Could you check a few things on this model? Use its own coordinates, in mm. A direction names the side the tool comes from. Coordinates: 2 decimals unless noted, no trailing zeros. Write each loop counter-clockwise with the first axis right and the second up, starting at its lowest first coordinate (ties: lowest second). Pieces come first, ordered by that corner, then holes.
Item 1: I want a section at C-C on x = -6.5. Please give me the cut outline in (y, z).
Item 2: Thinking about a two-plate mould opening in Z: for faces 1 (the cylindrical face through (0.18, 148.5, 0.07)), 2 (the flat face through (0, 160, 0)), 3 (the cylindrical face through (-11.923, 78.88, -3.755)), which applies, +Z half, -Z half, draft (parallel to the pull), parting line (faces both ways), or undercut?
Item 3: Which directions (+Z, -Z, +X, -X, +Y, -Y) give clear straight access to the entire face, cutting with the end or side of a thin tool? Please do faces 4 (the cylindrical face through (-0.05, 4.06, -3.77)), 5 (the flat face through (0, 0, 0)).
Item 4: I want a section at A-A on z = 0. Please give me the cut outline in (x, y), then the cut area to 3 significant figures.
Item 5: For P1, Ø2, axis at x = 0, z = -5, coming from the -Y side; P2, Ø1, axis at y = 114.5, z = 6.5, coming from the +X side; P3, Ø2, axis at y = 83.5, z = 2.5, coming from the +X side, each with a flat end and sliding along its axis, tell me the tip position at first contact or that it passes through.
Item 6: I want a section at D-D on z = 8. Please give me the cut outline in (x, y), then the cut area to 3 significant figures.
Item 7: I want a section at B-B on y = 55. Please give me the cut outline in (x, z), then the cut area to 3 significant figures.
Item 8: If I drill on probe 1 along Z at (x, y) = (0, 4.75); probe 2 along Y at (x, z) = (2.25, 0); probe 3 along Y at (x, z) = (-6.25, -1), over which ranges is the centre line in solid material (lowest first)?
Autodesk Inventor part; units mm, degrees
ref_plane "YZ Plane" through (0, 0, 0) normal (1, 0, 0) x (0, 1, 0)
ref_plane "XZ Plane" through (0, 0, 0) normal (0, 1, 0) x (-1, 0, 0)
ref_plane "XY Plane" through (0, 0, 0) normal (0, 0, 1) x (1, 0, 0)
sketch "Эскиз1" plane through (0, 0, 0) normal (0, 1, 0) x (-1, 0, 0)
  circle A0 centre (0, 0) radius 12.5
  dimension "d0" = 25
extrude "Выдавливание1" add sketch "Эскиз1" along normal blind 160
sketch "Эскиз2" plane through (0, 0, 0) normal (0, -1, 0) x (1, 0, 0)
  circle A0 centre (0, 0) radius 22.5
  line L0 (0, 0) -> (0, 5)
  line L1 (0, 0) -> (0, -5)
  dimension "d3" = 45
  dimension "d4" = 5
  dimension "d5" = 5
hole "Отверстие1" at (0, 0, 5) at (0, 0, -5) direction (0, 1, 0) diameter 2.459 depth 8 tip angle 118
sketch "Эскиз4" plane through (0, 0, 0) normal (1, 0, 0) x (0, 1, 0)
  line L0 (160, -12.5) -> (160, 12.5)
  line L1 (160, 0) -> (150, 0)
  circle A0 centre (150, 0) radius 1.5
  line L2 (160, 0) -> (150, 0)
  line L3 (150, 0) -> (155, 0)
  circle A1 centre (145, 0) radius 1.5
  line L4 (0, 0) -> (50, 0)
  circle A2 centre (50, 0) radius 1.5
  dimension "d30" = 3
  dimension "d35" = 10
  dimension "d49" = 50
  dimension "d50" = 3
extrude "Выдавливание3" cut sketch "Эскиз4" along normal mid plane 30.75 contours A0 | A2
thread "Резьба4"
thread "Резьба5"
properties part number "17701729.303788.008"
Response values:
1. outline: (0, -10.68) - (160, -10.68) - (160, 10.68) - (0, 10.68) - close; hole circle Ø3 at (50, 0); hole circle Ø3 at (150, 0)
2. face 1: undercut
2. face 2: draft
2. face 3: parting line
3. face 4: -Y
3. face 5: +Z, -Z, +X, -X, -Y
4. outline: (-12.5, 0) - (12.5, 0) - (12.5, 48.5) - (-12.5, 48.5) - close; (-12.5, 51.5) - (12.5, 51.5) - (12.5, 148.5) - (-12.5, 148.5) - close; (-12.5, 151.5) - (12.5, 151.5) - (12.5, 160) - (-12.5, 160) - close
4. area: 3,850 mm2
5. P1: stops at y = 8.14
5. P2: stops at x = 10.97
5. P3: stops at x = 12.41
6. outline: (-9.6, 0) - (9.6, 0) - (9.6, 160) - (-9.6, 160) - close
6. area: 3,070 mm2
7. outline: circle Ø25 at (0, 0)
7. area: 491 mm2
8. probe 1: z = -12.5 to -6.23, -3.77 to 3.77, 6.23 to 12.5
8. probe 2: y = 0 to 48.5, 51.5 to 148.5, 151.5 to 160
8. probe 3: y = 0 to 48.88, 51.12 to 148.88, 151.12 to 160
